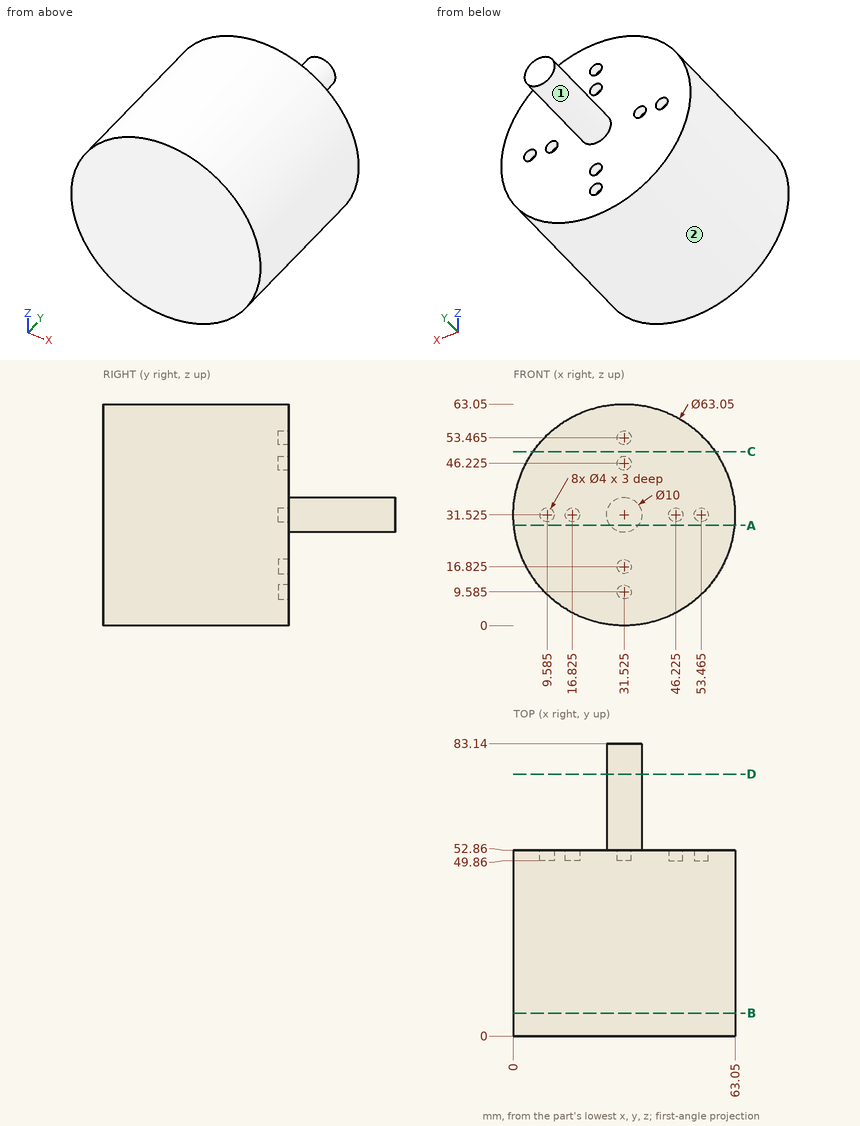
Geometry: see drawing. Coordinates: mm, zero at the bounding-box minimum. A direction names the side the tool comes from. Give positions to 0.01 mm unless a question says otherwise; leave off trailing zeros. Loops run counter-clockwise (first coordinate to the right, second up) from the corner with the lowest first, then second, coordinate; pieces in that order, holes last. Notation, with made-up numbers: (74, -11) -> (100, -11) arc R6 ccw to (100, 0) -> close; hole circle Ø1 at (62, 57). An arc over 180 degrees is marked (long way). Use CSV: the item, a comma, the result in double quotes.
(1) Cut plane D-D (y = 74.5). Output: boundary loops of the cut face in (x, z) (3 decimals).
From the geometry:
outline,"circle Ø10 at (31.525, 31.525)"
(2) Cut plane C-C (z = 49.5). Output: boundary loops of the cut face in (x, y).
From the geometry:
outline,"(5.63, 0) -> (57.42, 0) -> (57.42, 52.86) -> (5.63, 52.86) -> close"
(3) First-contact query: P1, Ø6.5, axis at x = 16.825, z = 31.525, coming from the +Y side; P2, Ø4, axis at y = 40.5, z = 53.5, coming from the +X side; P3, Ø4, axis at x = 44, y = 41, coming from the -Z side; P4, Ø4.5, axis at x = 31.525, z = 9.585, coming from the -Y side. Flat tips, straight axial feed; report the tip coordinate or a pass-through.
From the geometry:
P1,"y = 52.86"
P2,"x = 55.91"
P3,"z = 1.79"
P4,"y = 0"
(4) Cut plane A-A (z = 28.5). Output: boundary loops of the cut face in (x, y), plus the area to 3 significant figures.
From the geometry:
outline,"(0.15, 0) -> (62.9, 0) -> (62.9, 52.86) -> (35.51, 52.86) -> (35.51, 83.14) -> (27.54, 83.14) -> (27.54, 52.86) -> (0.15, 52.86) -> close"
area,"3,560 mm^2"
(5) Ray query, line 1 along Y through (x, z) = (3.5, 20); line 2 along X through (y, z) = (40, 30.5); line 3 along X through (y, z) = (36, 7). Return the intervals inside material, ascending. Write a range as [from, to].
From the geometry:
line 1,"[0, 52.86]"
line 2,"[0.02, 63.03]"
line 3,"[11.72, 51.33]"
(6) Cut plane B-B (y = 6.5). Output: boundary loops of the cut face in (x, z) (3 decimals).
From the geometry:
outline,"circle Ø63.05 at (31.525, 31.525)"
(7) Access query for the marked faces 1 and 2. Directions: +Z, -Z, +X, -X, +Y, -Y. A direction counts if a zero-diameter tool reaches every point of the face in a straight line with its end or side. Return the directions, or none.
From the geometry:
face 1,"+Y"
face 2,"+Y, -Y"
